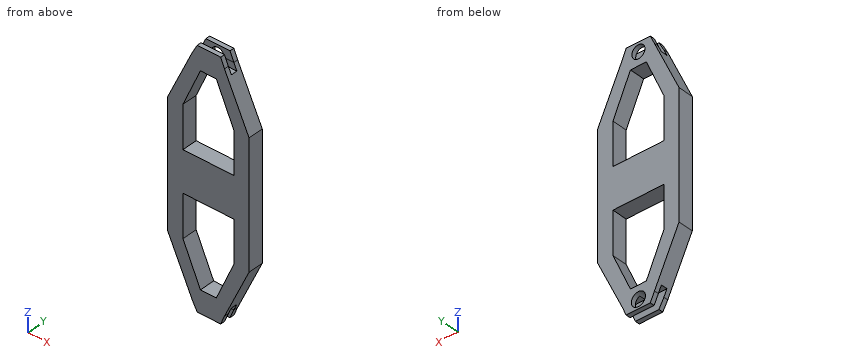
Autodesk Inventor part; units mm, degrees
ref_plane "YZ Plane" through (0, 0, 0) normal (1, 0, 0) x (0, 1, 0)
ref_plane "XZ Plane" through (0, 0, 0) normal (0, 1, 0) x (-1, 0, 0)
ref_plane "XY Plane" through (0, 0, 0) normal (0, 0, 1) x (1, 0, 0)
sketch "Sketch1" plane through (0, 0, 0) normal (0, 1, 0) x (-1, 0, 0)
  line L0 (0, -213.8682) -> (0, 213.8682)
  line L1 (20.1057, -144) -> (-20.1057, -144)
  line L2 (-50.827, -78.2337) -> (-50.827, 78.2337)
  line L3 (-20.1057, 144) -> (20.1057, 144)
  line L4 (50.773, 78.2337) -> (50.773, -78.2337)
  line L5 (158.1712, 0) -> (-85.66, 0)
  line L6 (50.773, 78.2337) -> (20.1057, 144)
  line L7 (50.773, 78.2337) -> (123.3381, 78.2337) construction
  line L8 (-50.827, 78.2337) -> (-20.1057, 144)
  line L9 (-20.1057, 144) -> (20.1057, 144)
  line L10 (31.723, 78.2337) -> (31.723, -78.2337)
  line L11 (-31.777, -78.2337) -> (-31.777, 78.2337)
  line L12 (-20.1057, -144) -> (20.1057, -144)
  line L13 (50.773, -78.2337) -> (20.1057, -144)
  line L14 (-50.827, -78.2337) -> (-20.1057, -144)
  line L15 (31.723, -25.4) -> (31.723, 25.4)
  line L16 (31.723, -25.4) -> (-31.777, -25.4)
  line L17 (31.723, 25.4) -> (-31.777, 25.4)
  line L18 (31.723, 78.2337) -> (9.9071, 127.5128)
  line L19 (-31.777, 78.2337) -> (-9.9611, 127.5128)
  line L20 (-9.9611, 127.5128) -> (9.9071, 127.5128)
  line L21 (50.773, 78.2337) -> (31.723, 78.2337)
  line L22 (-31.777, 78.2337) -> (-50.827, 78.2337)
  line L23 (31.723, -78.2337) -> (9.9071, -127.5128)
  line L24 (-31.777, -78.2337) -> (-9.9611, -127.5128)
  line L25 (-9.9611, -127.5128) -> (9.9071, -127.5128)
  line L26 (50.773, -78.2337) -> (31.723, -78.2337)
  line L27 (-31.777, -78.2337) -> (-50.827, -78.2337)
  point P0 (50.8, -140)
  point P1 (-50.8, 140)
  point P2 (-50.8, -140)
  dimension "d49" = 280
  dimension "d51" = 115
  dimension "d52" = 101.6
  dimension "d53" = 50.8
  dimension "d71" = 288
extrude "Extrusion1" add sketch "Sketch1" along normal blind 19.05 contours L1 L14 L27 L24 L25 L0 | L0 L25 L23 L26 L13 L1 | L16 L11 L5 L0 | L0 L5 L10 L16 | L26 L10 L5 L4 | L2 L5 L11 L27 | L5 L11 L17 L0 | L0 L17 L10 L5 | L5 L10 L21 L4 | L2 L22 L11 L5 | L21 L18 L20 L0 L3 L6 | L8 L3 L0 L20 L19 L22
sketch "Sketch9" plane through (50.827, 0, 78.2337) normal (1, 0, 0) x (0, 0, -1)
  line L0 (-65.7663, 19.05) -> (0, 19.05)
  line L1 (-65.7663, 19.05) -> (-65.7663, 0)
  line L2 (-65.7663, 0) -> (-65.7663, 19.05)
  line L3 (-65.7663, 9.525) -> (-52.4585, 9.525)
  line L4 (-65.7663, 13.4938) -> (-65.7663, 5.5563)
  line L5 (-65.7663, 19.05) -> (-77.0693, 19.05)
  line L6 (-65.7663, 19.05) -> (-54.4633, 19.05) construction
  line L7 (-65.7663, 13.4938) -> (-77.0693, 13.4937)
  line L8 (-77.0693, 13.4937) -> (-77.0693, 19.05)
  line L9 (-65.7663, 19.05) -> (-65.7663, 13.4938)
  line L10 (78.2337, -3.81) -> (78.2337, 22.86)
  line L11 (222.2337, 19.05) -> (233.5367, 19.05)
  line L12 (222.2337, 13.4938) -> (233.5367, 13.4937)
  line L13 (233.5367, 13.4937) -> (233.5367, 19.05)
  line L14 (222.2337, 19.05) -> (222.2337, 13.4938)
  point P0 (78.2337, 0)
  dimension "d55" = 7.9375
  dimension "d56" = 11.303
  dimension "d57" = 180
extrude "Extrusion9" add sketch "Sketch9" against normal up to surface (70.9326 mm away)
sketch "Sketch10" plane through (0, 19.05, 0) normal (0, 1, 0) x (1, 0, 0)
  line L0 (20.1057, -144) -> (50.827, -78.2337)
  line L1 (20.1057, -144) -> (15.3607, -155.303)
  line L2 (50.827, -155.303) -> (-20.1057, -155.303)
  line L3 (15.3607, -155.303) -> (50.53, -155.303)
  line L4 (50.827, -144) -> (20.1057, -144)
  line L5 (20.1057, -144) -> (50.827, -144)
  line L6 (50.827, -144) -> (50.827, -155.303)
  line L7 (50.827, -144) -> (50.827, -155.303)
  line L8 (50.827, -155.303) -> (50.827, -144)
  line L9 (50.827, -155.303) -> (15.3607, -155.303)
  line L10 (-71.093, 0) -> (71.147, 0)
  line L11 (20.1057, 144) -> (15.3607, 155.303)
  line L12 (15.3607, 155.303) -> (50.53, 155.303)
  line L13 (50.827, 144) -> (20.1057, 144)
  line L14 (20.1057, 144) -> (50.827, 144)
  line L15 (50.827, 144) -> (50.827, 155.303)
  line L16 (50.827, 144) -> (50.827, 155.303)
  line L17 (50.827, 155.303) -> (50.827, 144)
  line L18 (50.827, 155.303) -> (15.3607, 155.303)
  line L19 (-20.1057, -144) -> (-14.8343, -155.303)
  line L20 (-20.1057, -155.303) -> (-14.8343, -155.303)
  line L21 (-50.773, -78.2337) -> (-20.1057, -144)
  line L22 (-20.1057, -155.303) -> (-20.1057, -144)
  line L23 (-20.1057, 144) -> (-14.8343, 155.303)
  line L24 (-20.1057, 155.303) -> (-14.8343, 155.303)
  line L25 (-20.1057, 155.303) -> (-20.1057, 144)
  point P0 (0, 0)
extrude "Extrusion10" cut sketch "Sketch10" against normal up to surface (19.05 mm away)
sketch "Sketch11" plane through (50.827, 0, 78.2337) normal (1, 0, 0) x (0, 0, -1)
  line L0 (-65.7663, 0) -> (-65.7663, 13.4938)
  line L1 (-65.7663, 0) -> (-77.0693, 0)
  line L2 (-77.0693, 0) -> (-77.0693, 5.5626)
  line L3 (-77.0693, 5.5626) -> (-65.7663, 5.5626)
  line L4 (-77.0693, 19.05) -> (-65.7663, 19.05)
  line L5 (78.2337, -3.81) -> (78.2337, 22.86)
  line L6 (222.2337, 0) -> (233.5367, 0)
  line L7 (233.5367, 0) -> (233.5367, 5.5626)
  line L8 (233.5367, 5.5626) -> (222.2337, 5.5626)
  line L9 (222.2337, 0) -> (222.2337, 13.4938)
  line L10 (222.2337, 5.5626) -> (222.2337, 0)
  point P0 (78.2337, 0)
  dimension "d63" = 5.5626
  dimension "d76" = 11.303
extrude "Extrusion11" add sketch "Sketch11" against normal up to surface (70.9326 mm away)
sketch "Sketch12" plane through (50.827, 5.5626, -144) normal (0, 1, 0) x (1, 0, 0)
  line L0 (-70.9326, 11.303) -> (-70.9326, 0)
  line L1 (-70.9326, 11.303) -> (-70.9326, 0)
  line L2 (-70.9326, 0) -> (-64.7758, 11.303)
  line L3 (-64.7758, 11.303) -> (-70.9326, 11.303)
  line L4 (-35.4663, 11.303) -> (-65.6612, 11.303)
  line L5 (-35.4663, 11.303) -> (-30.7213, 0)
  line L6 (0, 0) -> (0, 11.303)
  line L7 (-30.7213, 0) -> (0, 0)
  line L8 (0, 0) -> (0, 11.303)
  line L9 (0, 11.303) -> (-35.4663, 11.303)
  line L10 (-121.92, -144) -> (20.32, -144)
  line L11 (-70.9326, -299.303) -> (-70.9326, -288)
  line L12 (-70.9326, -299.303) -> (-70.9326, -288)
  line L13 (-70.9326, -288) -> (-64.7758, -299.303)
  line L14 (-64.7758, -299.303) -> (-70.9326, -299.303)
  line L15 (-35.4663, -299.303) -> (-65.6612, -299.303)
  line L16 (-35.4663, -299.303) -> (-30.7213, -288)
  line L17 (0, -288) -> (0, -299.303)
  line L18 (-30.7213, -288) -> (0, -288)
  line L19 (0, -288) -> (0, -299.303)
  line L20 (0, -299.303) -> (-35.4663, -299.303)
  point P0 (-50.827, -144)
extrude "Extrusion12" cut sketch "Sketch12" against normal through all
sketch "Sketch13" plane through (0, 19.05, 0) normal (0, 1, 0) x (1, 0, 0)
  circle A0 centre (0, -144) radius 8.1915
  circle A1 centre (0, 144) radius 8.763
  line L0 (-71.093, 0) -> (71.147, 0)
  point P0 (0, 0)
  dimension "d68" = 16.383
  dimension "d69" = 17.526
  dimension "d70" = 288
extrude "Extrusion13" cut sketch "Sketch13" against normal up to surface (13.4874 mm away)
sketch "Sketch14" plane through (50.827, 0, 78.2337) normal (1, 0, 0) x (0, 0, -1)
  line L0 (-57.5748, 19.05) -> (-57.5748, 5.5626)
  line L1 (-57.5748, 19.05) -> (-57.5748, 5.5626)
  line L2 (-57.5748, 19.05) -> (-57.5748, 5.5626)
  line L3 (-65.7663, 13.4938) -> (-57.5748, 13.4938)
  line L4 (-57.5748, 5.5626) -> (-57.5748, 13.4938)
  line L5 (-65.7663, 5.5626) -> (-65.7663, 13.4938)
  line L6 (-57.5748, 5.5626) -> (-65.7663, 5.5626)
  line L7 (78.2337, -3.81) -> (78.2337, 22.86)
  line L8 (222.2337, 13.4938) -> (214.0422, 13.4938)
  line L9 (214.0422, 5.5626) -> (214.0422, 13.4938)
  line L10 (222.2337, 5.5626) -> (222.2337, 13.4938)
  line L11 (214.0422, 5.5626) -> (222.2337, 5.5626)
  point P0 (78.2337, 0)
extrude "Extrusion14" cut sketch "Sketch14" against normal through all
properties part number "Diff_BarV2"
Here's how the part is built. I have some questions about the finished solid (model axes, mm). Round coordinates to 2 decimals unless told otherwise and drop trailing zeros. Loops run counter-clockwise (first coordinate to the right, second up) from the corner with the lowest first, then second, coordinate; pieces in that order, holes last. Notation, with made-up numbers: (73, -12.5) -> (118, -12.5) arc R34 ccw to (118, 22.5) -> close; hole circle Ø4 at (-31.75, -9). An arc over 180 degrees is marked (long way). Answer as CSV lines item,"result".
1. If I drill on L1, parallel to Z at x = 0, y = 15.25; L2, parallel to X at y = 2.25, z = 29.5; L3, parallel to X at y = 17, z = 144, over which ranges is the centre line in solid material (lowest first)?
Final values:
L1,"z = -155.3 to -152.76, -135.24 to -127.51, -25.4 to 25.4, 127.51 to 135.81, 152.19 to 155.3"
L2,"x = -50.77 to -31.72, 31.78 to 50.83"
L3,"x = -20.11 to -8.19, 8.19 to 20.11"
2. If we section it at C-C on z = -106: Please give me the cut outline in (x, y).
Final values:
outline,"(-37.83, 0) -> (-19.43, 0) -> (-19.43, 19.05) -> (-37.83, 19.05) -> close; (19.48, 0) -> (37.86, 0) -> (37.86, 19.05) -> (19.48, 19.05) -> close"
3. If we section it at A-A on z = 52: Please give me the cut outline in (x, y).
Final values:
outline,"(-50.77, 0) -> (-31.72, 0) -> (-31.72, 19.05) -> (-50.77, 19.05) -> close; (31.78, 0) -> (50.83, 0) -> (50.83, 19.05) -> (31.78, 19.05) -> close"
4. If we section it at B-B on x = -28.5: Please give me the cut outline in (y, z).
Final values:
outline,"(0, -126) -> (19.05, -126) -> (19.05, -85.51) -> (0, -85.51) -> close; (0, -25.4) -> (19.05, -25.4) -> (19.05, 25.4) -> (0, 25.4) -> close; (0, 85.51) -> (19.05, 85.51) -> (19.05, 126) -> (0, 126) -> close"
5. If we section it at D-D on z = 131: Please give me the cut outline in (x, y).
Final values:
outline,"(-26.17, 0) -> (26.18, 0) -> (26.18, 19.05) -> (-26.17, 19.05) -> close"
6. For pin 1 (2.5 mm diameter, centred on x = 8, z = 139, fed in from -Y); pin 2 (4 mm diameter, centred on x = -15.5, y = 8, fed in from -Z); pin 3 (4 mm diameter, centred on y = 8, z = 114, fed in from +X); pin 4 (8 mm diameter, centred on x = 35.5, y = 7.5, fed in from -Z), each with a flat end and sliding along its axis, tell me the tip position at first contact or that it passes through.
Final values:
pin 1,"stops at y = 0"
pin 2,"stops at z = -135.81"
pin 3,"stops at x = 35.05"
pin 4,"stops at z = -119.61"
